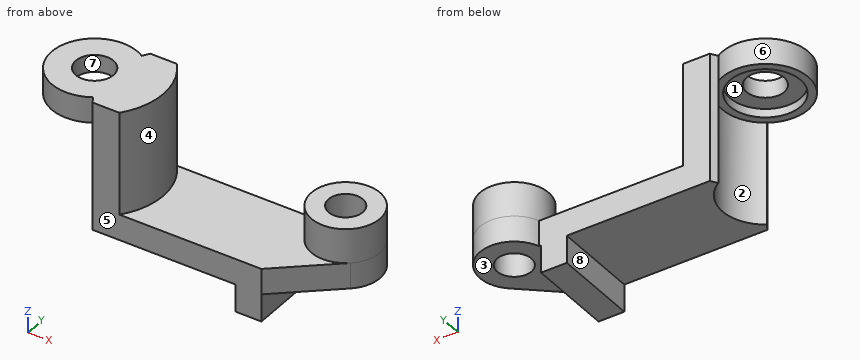
from build123d import *

# Parameters (mm, degrees)
SKETCH1_R           = 2.5
SKETCH1_R_2         = 1.1
BOSS_EXTRUDE1_DEPTH = 1
SKETCH2_R           = 2.5
SKETCH2_R_2         = 2.05
BOSS_EXTRUDE2_DEPTH = 0.5
BOSS_EXTRUDE4_DEPTH = 7.5
SKETCH5_R           = 1
BOSS_EXTRUDE5_DEPTH = 1.5
SKETCH6_W           = 1.5
SKETCH6_H           = 5
BOSS_EXTRUDE6_DEPTH = 1.6
SKETCH7_R           = 2
SKETCH7_R_2         = 1
BOSS_EXTRUDE7_DEPTH = 2


with BuildPart() as part:
    # Sketch1 → Boss-Extrude1 (new body)
    with BuildSketch(Plane.XY):
        Circle(SKETCH1_R)
        Circle(SKETCH1_R_2, mode=Mode.SUBTRACT)
    extrude(amount=-BOSS_EXTRUDE1_DEPTH)

    # Sketch2 → Boss-Extrude2 (add)
    with BuildSketch(Plane.XY.offset(-1)):
        Circle(SKETCH2_R)
        Circle(SKETCH2_R_2, mode=Mode.SUBTRACT)
    extrude(amount=-BOSS_EXTRUDE2_DEPTH)

    # Sketch3 → Boss-Extrude4 (add)
    with BuildSketch(Plane.XY):
        with BuildLine():
            Line((3.122498999, -2.5), (1.5612495, -2.5))
            Line((1.5612495, -2.5), (1.324234542, -2.120472324))
            ThreePointArc((1.324234542, -2.120472324), (2.5, 0), (1.324234542, 2.120472324))
            Line((1.324234542, 2.120472324), (1.5612495, 2.5))
            Line((1.5612495, 2.5), (3.122498999, 2.5))
            ThreePointArc((3.122498999, 2.5), (4, 0), (3.122498999, -2.5))
        make_face()
    extrude(amount=-BOSS_EXTRUDE4_DEPTH)

    # Sketch5 → Boss-Extrude5 (add)
    with BuildSketch(Plane(origin=(0, 0, -7.5), x_dir=(-1, 0, 0), z_dir=(0, 0, -1))):
        with BuildLine():
            Line((-3.122498999, -2.5), (-11.4, -2.5))
            Line((-11.4, -2.5), (-14.699339628, 0.319566992))
            ThreePointArc((-14.699339628, 0.319566992), (-14.529243579, 3.49069953), (-11.512038136, 2.5))
            Line((-11.512038136, 2.5), (-3.122498999, 2.5))
            Line((-3.122498999, 2.5), (-3.122498999, -2.5))
        make_face()
        with Locations((-13.4, 1.84)):
            Circle(SKETCH5_R, mode=Mode.SUBTRACT)
    extrude(amount=-BOSS_EXTRUDE5_DEPTH)

    # Sketch6 → Boss-Extrude6 (add)
    with BuildSketch(Plane(origin=(0, 0, -7.5), x_dir=(-1, 0, 0), z_dir=(0, 0, -1))):
        with Locations((-10.65, 0)):
            Rectangle(SKETCH6_W, SKETCH6_H)
    extrude(amount=BOSS_EXTRUDE6_DEPTH)

    # Sketch7 → Boss-Extrude7 (add)
    with BuildSketch(Plane.XY.offset(-6)):
        with Locations(Location((13.4, 1.84, 0), (0, 0, 160.731224509))):
            Circle(SKETCH7_R)
        with Locations(Location((13.4, 1.84, 0), (0, 0, 180))):
            Circle(SKETCH7_R_2, mode=Mode.SUBTRACT)
    extrude(amount=BOSS_EXTRUDE7_DEPTH)


solid = part.part
Can you work these out from the model? Positions are in its coordinate system, mm. Face numbers are marked on the shaded views. A direction names the side the tool comes from. Round coordinates to 2 decimals unless told otherwise and drop trailing zeros. Write each loop counter-clockwise with the first axis right and the second up, starting at its lowest first coordinate (ties: lowest second). Pieces come first, ordered by that corner, then holes. Notation, with made-up numbers: M 85.5,41 L 131.5,41 A10 cw 131.5,45 Z; hole C -31,-38.5 d4. An arc over 180 degrees is marked long. Use a Markdown table: item, result.
Item 1: I want a section at D-D (z = -6.75). List the corners of the cut face in (x, y) for me.
Found:
| item | result |
|---|---|
| outline | M 1.32,-2.12 L 1.56,-2.5 L 11.4,-2.5 L 14.7,0.32 A2 ccw long 11.51,2.5 L 1.56,2.5 L 1.32,2.12 A2.5 cw Z; hole C 13.4,1.84 d2 |
Item 2: For pin 1 Ø2.5 at (x, y) = (1, 1) entering from -Z; pin 2 Ø3.5 at (x, y) = (0, 0) entering from -Z; pin 3 Ø4.5 at (x, z) = (6, -4) entering from +Y; pin 4 Ø1.8 at (x, y) = (13.4, 1.84) entering from -Z, each with a flat end and sliding along its axis, tell me the tip position at first contact or that it passes through.
Found:
| item | result |
|---|---|
| pin 1 | stops at z = -7.5 |
| pin 2 | stops at z = -1 |
| pin 3 | stops at y = 2.5 |
| pin 4 | passes through |
Item 3: We'd pull the mould along Y, two halves only. Please class the marked faces 5, 6, 7 and 8: released by +Y, released by -Y, zero draft, split by the parting line, or undercut.
Found:
| item | result |
|---|---|
| face 5 | released by -Y |
| face 6 | split by the parting line |
| face 7 | undercut |
| face 8 | zero draft |
Item 4: I want a section at B-B (x = 0). List the corners of the cut face in (y, z) for me, and give its area (3 significant figures).
Found:
| item | result |
|---|---|
| outline | M -2.5,-1.5 L -2.05,-1.5 L -2.05,-1 L -1.1,-1 L -1.1,0 L -2.5,0 Z; M 1.1,-1 L 2.05,-1 L 2.05,-1.5 L 2.5,-1.5 L 2.5,0 L 1.1,0 Z |
| area | 3.25 mm2 |
Item 5: If I drill on line 1 along Y through (x, z) = (0, -1.25); line 2 along Z through (x, y) = (4, -1.5); line 3 along Z through (x, y) = (-1, -1), over which ranges is the centre line in solid material (lowest first)? Write a range as [from, to].
Found:
| item | result |
|---|---|
| line 1 | y = [-2.5, -2.05], [2.05, 2.5] |
| line 2 | z = [-7.5, -6] |
| line 3 | z = [-1, 0] |
Item 6: I want a section at A-A (z = -5.5). List the corners of the cut face in (x, y) for me, and give its area (3 significant figures).
Found:
| item | result |
|---|---|
| outline | M 1.32,-2.12 L 1.56,-2.5 L 3.12,-2.5 A4 ccw 3.12,2.5 L 1.56,2.5 L 1.32,2.12 A2.5 cw Z; C 13.4,1.84 d4; hole C 13.4,1.84 d2 |
| area | 17.8 mm2 |
Item 7: Which directions (+Z, -Z, +X, -X, +Y, -Y) give clear straight access to the entire face, cutting with the end or side of a thin tool? Please do the marked faces 1, 2, 3 and 4.
Found:
| item | result |
|---|---|
| face 1 | -Z |
| face 2 | -Z, -X |
| face 3 | -Z, +X, +Y, -Y |
| face 4 | +Z |
Item 8: I want a section at C-C (y = 1.5). List the corners of the cut face in (x, z) for me, and give its area (3 significant figures).
Found:
| item | result |
|---|---|
| outline | M -2,-1.5 L -1.4,-1.5 L -1.4,-1 L 1.4,-1 L 1.4,-1.5 L 2,-1.5 L 2,-7.5 L 9.9,-7.5 L 9.9,-9.1 L 11.4,-9.1 L 11.4,-7.5 L 12.46,-7.5 L 12.46,-4 L 11.43,-4 L 11.43,-6 L 3.71,-6 L 3.71,0 L -2,0 Z; M 14.34,-7.5 L 15.37,-7.5 L 15.37,-4 L 14.34,-4 Z |
| area | 38.6 mm2 |
